```python
from build123d import *

# Parameters (mm, degrees)
F0_R     = 19.609183
F0_W     = 10.1
F0_H     = 3.1
F1_DEPTH = 3
F2_DEPTH = 13


with BuildPart() as f1:
    # F0 (on Top) → F1 (new body)
    with BuildSketch(Plane.XY):
        Circle(F0_R)
        Polygon((-12.493552, -12.409452), (-16.993677, 4.615007), (-4.500125, 17.024459), (12.493552, 12.409452), (16.993677, -4.615007), (4.500125, -17.024459), align=None, mode=Mode.SUBTRACT)
        Polygon((-4.500125, 17.024459), (-16.993677, 4.615007), (-12.493552, -12.409452), (4.500125, -17.024459), (16.993677, -4.615007), (12.493552, 12.409452), align=None)
        Rectangle(F0_W, F0_H, mode=Mode.SUBTRACT)
    extrude(amount=F1_DEPTH)

    # F0 (on Top) → F2 (join)
    with BuildSketch(Plane.XY):
        Circle(F0_R)
        Polygon((-12.493552, -12.409452), (-16.993677, 4.615007), (-4.500125, 17.024459), (12.493552, 12.409452), (16.993677, -4.615007), (4.500125, -17.024459), align=None, mode=Mode.SUBTRACT)
    extrude(amount=-F2_DEPTH)


solid = f1.part
```
The listing builds one solid part. Answer for the finished solid, in the listing's coordinates (mm). A direction names the side the tool comes from. Round coordinates to 2 decimals unless told otherwise and drop trailing zeros. Loops run counter-clockwise (first coordinate to the right, second up) from the corner with the lowest first, then second, coordinate; pieces in that order, holes last.
1) A cutting plane is placed at B-B on z = -1.25. Determine the outline of the cut face in (x, y) (3 decimals).
Outcome:
outline: circle Ø39.218 at (0, 0); hole (-16.994, 4.615) - (-12.494, -12.409) - (4.5, -17.024) - (16.994, -4.615) - (12.494, 12.409) - (-4.5, 17.024) - close
2) A cutting plane is placed at D-D on y = -15.5. Determine the outline of the cut face in (x, z), plus the area to 3 significant figures.
Outcome:
outline: (-12.01, -13) - (-1.11, -13) - (-1.11, 0) - (6.03, 0) - (6.03, -13) - (12.01, -13) - (12.01, 3) - (-12.01, 3) - close
area: 291 mm2
3) Given P1, Ø3, axis at x = 4, y = -4, coming from the -Z side; P2, Ø8, axis at y = 2.5, z = -4, coming from the +X side; P3, Ø2.5, axis at x = 0.5, z = 2, coming from the +Y side; P4, Ø2.5, axis at x = -1, z = 2, coming from the -Y side, each flat-ended and moving along its own axis, determine where each tip first touches the part or whether it passes through.
Outcome:
P1: stops at z = 0
P2: stops at x = 19.61
P3: stops at y = 19.61
P4: stops at y = -19.61
4) Consider line 1 (Z direction, x = 1, y = -14); line 2 (Y direction, x = -2.5, z = -6.5); line 3 (X direction, y = -9.5, z = -9.5). Determine where each line is inside the solid, lowest interval first.
Outcome:
line 1: z = 0 to 3
line 2: y = -19.45 to -15.12, 16.48 to 19.45
line 3: x = -17.15 to -13.26, 12.08 to 17.15
5) A cutting plane is placed at A-A on y = 0. Determine the outline of the cut face in (x, z).
Outcome:
outline: (-19.61, -13) - (-15.77, -13) - (-15.77, 0) - (-5.05, 0) - (-5.05, 3) - (-19.61, 3) - close; (5.05, 0) - (15.77, 0) - (15.77, -13) - (19.61, -13) - (19.61, 3) - (5.05, 3) - close
6) For a pull along Y with two mould halves and no side action, classify faces 1 (the face through (0, -4, 3)), 2 (the face through (-4.251, -19.143, -4.888)), 3 (the face through (0, 4, 0)), 4 (the face through (14.71, 4.02, -6.41)) as released by +Y, released by -Y, zero draft, split by the parting line, or undercut.
Outcome:
face 1: zero draft
face 2: split by the parting line
face 3: undercut
face 4: undercut
7) For faces 5 (the face through (3.88, 14.75, -6.41)), 6 (the face through (-5.05, 0, 1)), 7 (the face through (6, 15, -13)), determine the directions among +Z, -Z, +X, -X, +Y, -Y from which every point of the face is accessible in a straight line to the end or side of a thin tool.
Outcome:
face 5: -Z
face 6: +Z, -Z
face 7: -Z, +X, -X, +Y, -Y
8) A cutting plane is placed at C-C on x = 0. Determine the outline of the cut face in (y, z).
Outcome:
outline: (-19.61, -13) - (-15.8, -13) - (-15.8, 0) - (-1.55, 0) - (-1.55, 3) - (-19.61, 3) - close; (1.55, 0) - (15.8, 0) - (15.8, -13) - (19.61, -13) - (19.61, 3) - (1.55, 3) - close
